Read the model definition and answer for the solid it produces. Units are mm, in the model's axes. A direction names the side the tool comes from. Coordinates: 2 decimals unless noted, no trailing zeros. Write each loop counter-clockwise with the first axis right and the second up, starting at its lowest first coordinate (ties: lowest second). Pieces come first, ordered by that corner, then holes.
Item 1: A tool of negligible diameter and unlimited length cuts with its end or side. For faces 4 (the face through (8.523, -0.993, -0.913)), 5 (the face through (0, -1.5, 0)), from which of +Z, -Z, +X, -X, +Y, -Y can it reach the whole face along a straight path? Write none if from no direction.
Item 2: Section A-A (z = -19) is taken. Give the vertices of the cut face in (x, y), then the cut area to 3 significant figures.
Item 3: Determine the mould class of faces 1 (the face through (23.846, -0.021, 7.509)), 2 (the face through (-8.51, -0.99, -1.41)), 3 (the face through (22.1, -1.5, -7.3)) for opening direction X: released by +X, released by -X, zero draft, split by the parting line, or undercut.
Item 4: Section B-B (x = -3) is taken. Give the vertices of the cut face in (y, z), then the cut area to 3 significant figures.
Item 5: Each of these flat-tipped pins is pushed along its axis until it touches: P1, Ø1.5, axis at x = 1, y = -0.5, coming from the +Z side; P2, Ø10, axis at x = 16.5, z = -1, coming from the -Y side. Where does it stop, or does it pass through?
Item 6: Straight lines are drawn through the part: probe 1 along X at (y, z) = (-1.2, 4.5); probe 2 along Z at (x, y) = (0, -0.95); probe 3 along Y at (x, z) = (22, 4). For each, find the intervals that lie inside material, in ascending order.
Item 7: Section D-D (x = -20.5) is taken. Give the vertices of the cut face in (y, z), then the cut area to 3 significant figures.
Item 8: Section C-C (y = 0.15) is taken. Give the vertices of the cut face in (x, z), then the cut area to 3 significant figures.
from build123d import *

# Parameters (mm, degrees)
F0_R     = 25
F1_DEPTH = 1.5
F2_R     = 23
F3_DEPTH = 1
F5_DEPTH = 1
F7_DEPTH = 1


with BuildPart() as f1:
    # F0 (on Front) → F1 (new body, symmetric)
    with BuildSketch(Plane.XZ):
        Circle(F0_R)
    extrude(amount=F1_DEPTH, both=True)

    # F2 (on face) → F3 (cut)
    with BuildSketch(Plane.XZ.offset(1.5)):
        Circle(F2_R)
    extrude(amount=-F3_DEPTH, mode=Mode.SUBTRACT)

    # F4 (on face) → F5 (join)
    with BuildSketch(Plane.XZ.offset(0.5)):
        Polygon((9.7037305963, 0.4278131442), (-0.2857921618, 9.9359199418), (-9.7544326689, -0.1756772261), (0.3401018036, -10.2059959115), align=None)
    extrude(amount=F5_DEPTH)

    # F6 (on face) → F7 (join)
    with BuildSketch(Plane.XZ.offset(0.5)):
        Polygon((7.3748351342, -2.2169979865), (2.7204787029, -7.5027198647), (9.2619833934, -8.3943828612), align=None)
        Polygon((-2.1856052259, -7.6963560187), (-7.2287256394, -2.6853171189), (-8.6267801345, -9.1355453032), align=None)
    extrude(amount=F7_DEPTH)


solid = f1.part
Established:
1. face 4: -Y
1. face 5: +Z, -Z, +X, -X, -Y
2. outline: (-16.25, -1.5) - (-12.96, -1.5) - (-12.96, -0.5) - (12.96, -0.5) - (12.96, -1.5) - (16.25, -1.5) - (16.25, 1.5) - (-16.25, 1.5) - close
2. area: 71.6 mm2
3. face 1: split by the parting line
3. face 2: undercut
3. face 3: zero draft
4. outline: (-1.5, -24.82) - (1.5, -24.82) - (1.5, 24.82) - (-1.5, 24.82) - (-1.5, 22.8) - (-0.5, 22.8) - (-0.5, 7.04) - (-1.5, 7.04) - (-1.5, -7.88) - (-0.5, -7.88) - (-0.5, -22.8) - (-1.5, -22.8) - close
4. area: 118 mm2
5. P1: stops at z = 25
5. P2: stops at y = -0.5
6. probe 1: x = -24.59 to -22.56, -5.38 to 5.43, 22.56 to 24.59
6. probe 2: z = -25 to -23, -9.87 to 9.66, 23 to 25
6. probe 3: y = -0.5 to 1.5
7. outline: (-1.5, -14.31) - (1.5, -14.31) - (1.5, 14.31) - (-1.5, 14.31) - (-1.5, 10.43) - (-0.5, 10.43) - (-0.5, -10.43) - (-1.5, -10.43) - close
7. area: 65.0 mm2
8. outline: circle Ø50 at (0, 0)
8. area: 1,960 mm2
